Work out the finished part from the listing and answer in its coordinate system (mm). A direction names the side the tool comes from. Round coordinates to 2 decimals unless told otherwise and drop trailing zeros. Order: outer loops, then holes, each group sorted by start corner. A loop starts at its lowest first (then second) coordinate and runs counter-clockwise, first axis right, second up. Notation, with made-up numbers: (19.25, 75.5) - (69.25, 75.5) arc R32 ccw to (69.25, 105.5) - close; hole circle Ø6 at (9, 67.25). An arc over 180 degrees is marked (long way). Answer in a Markdown table with one row per item.
from build123d import *

# Parameters (mm, degrees)
SKETCH2_R               = 2.1
SKETCH2_R_2             = 7.1
BOSS_EXTRUDE1_DEPTH     = 5
SKETCH3_R               = 7.6
CUT_EXTRUDE1_DEPTH      = 1
SKETCH4_R               = 2.1
CUT_EXTRUDE2_DEPTH      = 6
SKETCH5_R               = 4
CUT_EXTRUDE3_DEPTH      = 2.5
CUT_EXTRUDE4_DEPTH      = 6
CUT_EXTRUDE5_DEPTH      = 6
CUT_EXTRUDE6_DEPTH      = 1
CUT_EXTRUDE6_DEPTH_BACK = 6


with BuildPart() as part:
    # Sketch2 → Boss-Extrude1 (new body)
    with BuildSketch(Plane(origin=(0, 0, 0), x_dir=(1, 0, 0), z_dir=(0, 1, 0))):
        with BuildLine():
            Line((50, 60), (-52.5, 60))
            ThreePointArc((-52.5, 60), (-59.571067812, 57.071067812), (-62.5, 50))
            Line((-62.5, 50), (-62.5, -50))
            ThreePointArc((-62.5, -50), (-59.571067812, -57.071067812), (-52.5, -60))
            Line((-52.5, -60), (50, -60))
            ThreePointArc((50, -60), (57.071067812, -57.071067812), (60, -50))
            Line((60, -50), (60, 50))
            ThreePointArc((60, 50), (57.071067812, 57.071067812), (50, 60))
        make_face()
        with Locations((-38.25, -38.25)):
            Circle(SKETCH2_R, mode=Mode.SUBTRACT)
        with Locations((38.25, -38.25)):
            Circle(SKETCH2_R, mode=Mode.SUBTRACT)
        with Locations((-38.25, 38.25)):
            Circle(SKETCH2_R, mode=Mode.SUBTRACT)
        Circle(SKETCH2_R_2, mode=Mode.SUBTRACT)
        with Locations((38.25, 38.25)):
            Circle(SKETCH2_R, mode=Mode.SUBTRACT)
    extrude(amount=BOSS_EXTRUDE1_DEPTH)

    # Sketch3 → Cut-Extrude1 (cut)
    with BuildSketch(Plane(origin=(0, 5, 0), x_dir=(1, 0, 0), z_dir=(0, 1, 0))):
        Circle(SKETCH3_R)
    extrude(amount=-CUT_EXTRUDE1_DEPTH, mode=Mode.SUBTRACT)

    # Sketch4 → Cut-Extrude2 (cut, through all)
    with BuildSketch(Plane.XZ):
        with Locations((-40.988809693, -52)):
            Circle(SKETCH4_R)
        with Locations((-8.988809693, -52)):
            Circle(SKETCH4_R)
        with Locations((9.011190307, -52)):
            Circle(SKETCH4_R)
        with Locations((41.011190307, -52)):
            Circle(SKETCH4_R)
        with BuildLine():
            ThreePointArc((-43.088809693, 52), (-40.988809693, 49.9), (-38.888809693, 52))
            Line((-38.888809693, 52), (-43.088809693, 52))
        make_face()
        with BuildLine():
            Line((-43.088809693, 52), (-38.888809693, 52))
            ThreePointArc((-38.888809693, 52), (-40.988809693, 54.1), (-43.088809693, 52))
        make_face()
        with BuildLine():
            ThreePointArc((-6.888809693, 52), (-8.988809693, 54.1), (-11.088809693, 52))
            Line((-11.088809693, 52), (-6.888809693, 52))
        make_face()
        with BuildLine():
            Line((-6.888809693, 52), (-11.088809693, 52))
            ThreePointArc((-11.088809693, 52), (-8.988809693, 49.9), (-6.888809693, 52))
        make_face()
        with Locations((9.011190307, 52)):
            Circle(SKETCH4_R)
        with Locations((41.011190307, 52)):
            Circle(SKETCH4_R)
    extrude(amount=-CUT_EXTRUDE2_DEPTH, mode=Mode.SUBTRACT)

    # Sketch5 → Cut-Extrude3 (cut)
    with BuildSketch(Plane.XZ):
        with Locations((-38.25, 38.25)):
            Circle(SKETCH5_R)
        with Locations((38.25, 38.25)):
            Circle(SKETCH5_R)
        with Locations((38.25, -38.25)):
            Circle(SKETCH5_R)
        with Locations((-38.25, -38.25)):
            Circle(SKETCH5_R)
    extrude(amount=-CUT_EXTRUDE3_DEPTH, mode=Mode.SUBTRACT)

    # Sketch7 → Cut-Extrude4 (cut, through all)
    with BuildSketch(Plane.XZ):
        with BuildLine():
            Line((32, 18.1), (42, 18.1))
            ThreePointArc((42, 18.1), (44.1, 16), (42, 13.9))
            Line((42, 13.9), (32, 13.9))
            ThreePointArc((32, 13.9), (29.9, 16), (32, 18.1))
        make_face()
        with BuildLine():
            Line((32, -13.9), (42, -13.9))
            ThreePointArc((42, -13.9), (44.1, -16), (42, -18.1))
            Line((42, -18.1), (32, -18.1))
            ThreePointArc((32, -18.1), (29.9, -16), (32, -13.9))
        make_face()
    extrude(amount=-CUT_EXTRUDE4_DEPTH, mode=Mode.SUBTRACT)

    # Sketch8 → Cut-Extrude5 (cut, through all)
    with BuildSketch(Plane.XZ):
        with BuildLine():
            Line((-57, 18.1), (-26, 18.1))
            ThreePointArc((-26, 18.1), (-23.9, 16), (-26, 13.9))
            Line((-26, 13.9), (-57, 13.9))
            ThreePointArc((-57, 13.9), (-59.1, 16), (-57, 18.1))
        make_face()
        with BuildLine():
            Line((-57, -13.9), (-26, -13.9))
            ThreePointArc((-26, -13.9), (-23.9, -16), (-26, -18.1))
            Line((-26, -18.1), (-57, -18.1))
            ThreePointArc((-57, -18.1), (-59.1, -16), (-57, -13.9))
        make_face()
    extrude(amount=-CUT_EXTRUDE5_DEPTH, mode=Mode.SUBTRACT)

    # Sketch9 → Cut-Extrude6 (cut, two sides)
    with BuildSketch(Plane(origin=(0, 5, 0), x_dir=(1, 0, 0), z_dir=(0, 1, 0))) as cut_extrude6_sk:
        Polygon((0, -18.55416869), (-26.293557739, -29.33935049), (0, -43.78052612), (32.385143241, -29.33935049), align=None)
        Polygon((0, 43.78052612), (32.385143241, 29.33935049), (0, 18.55416869), (-26.293557739, 29.33935049), align=None)
    extrude(amount=CUT_EXTRUDE6_DEPTH, mode=Mode.SUBTRACT)
    extrude(cut_extrude6_sk.sketch, amount=-CUT_EXTRUDE6_DEPTH_BACK, mode=Mode.SUBTRACT)


solid = part.part
1) Find section B-B, the plane z = 52. Give the vertices of the cut face in (x, y), then the cut area to 3 significant figures.
Filled in:
| item | result |
|---|---|
| outline | (-62.3, 0) - (-43.09, 0) - (-43.09, 5) - (-62.3, 5) - close; (-38.89, 0) - (-11.09, 0) - (-11.09, 5) - (-38.89, 5) - close; (-6.89, 0) - (6.91, 0) - (6.91, 5) - (-6.89, 5) - close; (11.11, 0) - (38.91, 0) - (38.91, 5) - (11.11, 5) - close; (43.11, 0) - (59.8, 0) - (59.8, 5) - (43.11, 5) - close |
| area | 526 mm^2 |
2) Find section C-C, the plane y = 1. Give the number of separate pieces and of enclosed holes in the cut face, then the cut area to 3 significant figures.
Filled in:
| item | result |
|---|---|
| separate pieces | 1 |
| enclosed holes | 19 |
| area | 12,300 mm^2 |
3) Find section A-A, the plane z = 16. Give the vertices of the cut face in (x, y).
Filled in:
| item | result |
|---|---|
| outline | (-62.5, 0) - (-59.1, 0) - (-59.1, 5) - (-62.5, 5) - close; (-23.9, 0) - (29.9, 0) - (29.9, 5) - (-23.9, 5) - close; (44.1, 0) - (60, 0) - (60, 5) - (44.1, 5) - close |
4) Find the intervals of material crossed by probe 1 along Z at (x, y) = (-38.25, 3.75); probe 2 along Z at (x, y) = (-48, 0.5); probe 3 along Z at (x, y) = (-38.25, 1.75), in increasing order. Write a range as from..to.
Filled in:
| item | result |
|---|---|
| probe 1 | z = -60..-40.35, -36.15..-18.1, -13.9..13.9, 18.1..36.15, 40.35..60 |
| probe 2 | z = -60..-18.1, -13.9..13.9, 18.1..60 |
| probe 3 | z = -60..-42.25, -34.25..-18.1, -13.9..13.9, 18.1..34.25, 42.25..60 |
5) Which of the six approach directions +Z, -Z, +X, -X, +Y, -Y give full straight-line access (tool end or side, diameter ignored) to faces 1 (the face through (37.729, 1.232, -34.284)), 2 (the face through (-7.593, 4.507, -0.334)), 3 (the face through (-12.96, 2.54, 23.87))?
Filled in:
| item | result |
|---|---|
| face 1 | -Y |
| face 2 | +Y |
| face 3 | +Y, -Y |
6) Find section D-D, the plane z = -21. Give the vertices of the cut face in (x, y).
Filled in:
| item | result |
|---|---|
| outline | (-62.5, 0) - (-5.96, 0) - (-5.96, 5) - (-62.5, 5) - close; (7.34, 0) - (60, 0) - (60, 5) - (7.34, 5) - close |
7) The mould has two halves that part along X. Classify faces 4 (the face through (-2, 0, 12)), 5 (the face through (56.99, 2.46, 57.15)), 6 (the face through (29.9, 2.5, 16)): released by +X, released by -X, zero draft, split by the parting line, or undercut.
Filled in:
| item | result |
|---|---|
| face 4 | zero draft |
| face 5 | released by +X |
| face 6 | undercut |
8) This flat-tipped pin is pushed along its axis until it touches: pin 1 (4 mm diameter, centred on x = 39.5, z = -38.5, fed in from -Y). Where does it stop, or does it pass through?
Filled in:
| item | result |
|---|---|
| pin 1 | stops at y = 2.5 |
